Can you work these out from the model? Positions are in its coordinate system, mm. A direction names the side the tool comes from. Give positions to 0.01 mm unless a question says otherwise; leave off trailing zeros. Write each loop counter-clockwise with the first axis right and the second up, starting at its lowest first coordinate (ties: lowest second). Pieces come first, ordered by that corner, then holes.
1. Suppose I cut it at D-D (z = 21). Please give me the cut outline in (x, y) (1 decimal).
2. Thinking about a two-plate mould opening in X: for faces 3 (the cylindrical face through (8.767, -16.856, 25.232)), 4 (the flat face through (-15, -12, 24)), 5 (the cylindrical face through (-9.5, 0.07, 13.95)), which applies, pulls with the +X half, pulls with the -X half, needs draft (parallel to the pull), parting line crosses it, or undercut?
3. Suppose I cut it at C-C (z = 15). Please give me the cut outline in (x, y) (1 decimal).
4. Suppose I cut it at A-A (x = 0). Please give me the cut outline in (y, z), and give its area (3 significant figures).
5. I'm going to push flat-ended pins straight in: pin 1 (3 mm diameter, centred on y = -5, z = 10.5, fed in from +X); pin 2 (4 mm diameter, centred on x = -0.5, z = 9.5, fed in from -Y); pin 3 (2 mm diameter, centred on x = -9.5, z = 17, fed in from -Y). Where does each tip first touch, or does it pass through?
6. On a 3-axis mill with a long thin cutter (end or side, diameter ignored), from which of +Z, -Z, +X, -X, +Y, -Y can I reach the whole of each face in a straight line? I mean faces 1 (the flat face through (0, 0, 10.5)), 2 (the flat face through (14, 9, 26.5)). Say none if no direction works.
7. If I drill on probe 1 along Z at (x, y) = (0.5, 4); probe 2 along Y at (x, z) = (-10.5, 17.5); probe 3 along X at (y, z) = (4, 11), over which ranges is the centre line in solid material (lowest first)?
8. Suppose I cut it at B-B (y = 0). Please give me the cut outline in (x, z), and give its area (3 significant figures).
```python
from build123d import *

# Parameters (mm, degrees)
F2_R     = 19
F3_DEPTH = 2.5
F6_R     = 3
F7_R     = 1.5
F8_DEPTH = 8.5
F9_R     = 1.5


with BuildPart() as f1:
    # F0 (on Front) → F1 (revolve)
    with BuildSketch(Plane.XZ):
        Polygon((0, 24), (0, 0), (17, 0), (22.5, 24), align=None)
    revolve(axis=Axis((0, 0, 12), (0, 0, 1)))

    # F2 (on face) → F3 (join)
    with BuildSketch(Plane.XY.offset(24)):
        Circle(F2_R)
    extrude(amount=F3_DEPTH)

    # F4 (on Front) → F5 (revolve, cut)
    with BuildSketch(Plane.XZ):
        Polygon((16.25, 26.5), (0, 26.5), (0, 10.5), (13.25, 10.5), align=None)
    revolve(axis=Axis((0, 0, 18.5), (0, 0, -1)), mode=Mode.SUBTRACT)

    # F6
    f6_edges = [f1.edges().sort_by_distance(p)[0] for p in [
        (-13.25, 0, 10.5),
    ]]
    fillet(f6_edges, radius=F6_R)

    # F7 (on face) → F8 (join)
    with BuildSketch(Plane.XY.offset(10.5)):
        with Locations((-8, 0)):
            Circle(F7_R)
        with Locations((6, 0)):
            Circle(F7_R)
    extrude(amount=F8_DEPTH)

    # F9
    f9_edges = [f1.edges().sort_by_distance(p)[0] for p in [
        (-9.5, 0, 19),
        (4.5, 0, 19),
    ]]
    fillet(f9_edges, radius=F9_R)


solid = f1.part
```
Checks:
1. outline: circle Ø43.6 at (0, 0); hole circle Ø30.4 at (0, 0)
2. face 3: parting line crosses it
2. face 4: needs draft
2. face 5: undercut
3. outline: circle Ø40.9 at (0, 0); circle Ø3 at (-8, 0); circle Ø3 at (6, 0); hole circle Ø28.2 at (0, 0)
4. outline: (-22.5, 24) - (-17, 0) - (17, 0) - (22.5, 24) - (19, 24) - (19, 26.5) - (16.25, 26.5) - (13.71, 12.95) arc R3 cw to (10.76, 10.5) - (-10.76, 10.5) arc R3 cw to (-13.71, 12.95) - (-16.25, 26.5) - (-19, 26.5) - (-19, 24) - close
4. area: 573 mm2
5. pin 1: stops at x = 19.25
5. pin 2: stops at y = -19.63
5. pin 3: stops at y = -19.15
6. face 1: +Z
6. face 2: +Z, +X, -X, +Y, -Y
7. probe 1: z = 0 to 10.5
7. probe 2: y = -18.2 to -10.09, 10.09 to 18.2
7. probe 3: x = -19.11 to -11.76, 11.76 to 19.11
8. outline: (-22.5, 24) - (-17, 0) - (17, 0) - (22.5, 24) - (19, 24) - (19, 26.5) - (16.25, 26.5) - (13.71, 12.95) arc R3 cw to (10.76, 10.5) - (7.5, 10.5) - (7.5, 17.5) arc R1.5 ccw to (4.5, 17.5) - (4.5, 10.5) - (-6.5, 10.5) - (-6.5, 17.5) arc R1.5 ccw to (-9.5, 17.5) - (-9.5, 10.5) - (-10.76, 10.5) arc R3 cw to (-13.71, 12.95) - (-16.25, 26.5) - (-19, 26.5) - (-19, 24) - close
8. area: 623 mm2
